```python
from build123d import *

# Parameters (mm, degrees)
SKETCH2_R               = 4.7625
BOSS_EXTRUDE1_DEPTH     = 75.565
CUT_EXTRUDE1_DEPTH      = 8.255
CUT_EXTRUDE1_DEPTH_BACK = 8.255
SKETCH3_OUTSIDE_W       = 26.878
SKETCH3_OUTSIDE_H       = 26.878
SKETCH3_OUTSIDE_R       = 4.1275


with BuildPart() as part:
    # Sketch2 → Boss-Extrude1 (new body)
    with BuildSketch(Plane(origin=(0, 0, 0), x_dir=(1, 0, 0), z_dir=(0, 1, 0))):
        with Locations(Location((0, 0, 0), (0, 0, 270))):
            Circle(SKETCH2_R)
    extrude(amount=BOSS_EXTRUDE1_DEPTH)

    # Sketch3 outside → Cut-Extrude1 (cut, two sides: drawn at the far end of the back side and taken through both)
    with BuildSketch(Plane(origin=(0, 37.7825, 0), x_dir=(1, 0, 0), z_dir=(0, 1, 0)).offset(-CUT_EXTRUDE1_DEPTH_BACK)):
        Rectangle(SKETCH3_OUTSIDE_W, SKETCH3_OUTSIDE_H)
        with Locations(Location((0, 0, 0), (0, 0, 270))):
            Circle(SKETCH3_OUTSIDE_R, mode=Mode.SUBTRACT)
    extrude(amount=CUT_EXTRUDE1_DEPTH + CUT_EXTRUDE1_DEPTH_BACK, mode=Mode.SUBTRACT)


solid = part.part
```
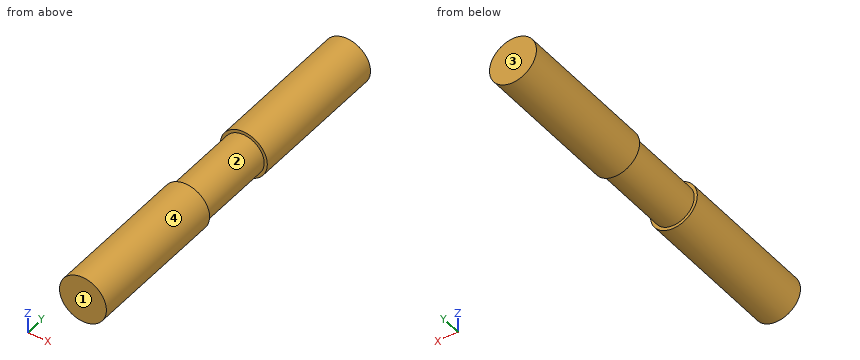
Geometry check sheet. Reference: the model listing, model coordinates, mm. Face numbers are marked on the shaded views. Give positions to 0.01 mm unless a question says otherwise; leave off trailing zeros. Loops run counter-clockwise (first coordinate to the right, second up) from the corner with the lowest first, then second, coordinate; pieces in that order, holes last. Notation, with made-up numbers: (51, -33.5) - (59, -33.5) arc R24 cw to (59, 2.5) - close; hole circle Ø1 at (66.25, 45.5). An arc over 180 degrees is marked (long way). Use CSV: the item, a comma, the result in double quotes. Start each with the question number.
Q1. Section check C-C, the plane y = 53. Record the cut outline in (x, z) (1 decimal), and give its area (3 significant figures).
Q2. Go/stop test with a flat-tipped pin: pin 1 Ø1.5 at (y, z) = (8, -2) entering from -X. Record where the tip stops, or that it passes through.
Q3. Release check for a two-part mould opening along Y. For the marked faces 1, 2, 3 and 4 record: +Y half, -Y half, draft (parallel to the pull), parting line (faces both ways), or undercut.
Q4. Section check B-B, the plane z = 0. Record the cut outline in (x, y) (1 decimal).
Q5. Scan lines: probe 1 along Y at (x, z) = (-3.75, 2) (1 decimal); probe 2 along Z at (x, y) = (-0.25, 5.5); probe 3 along Z at (x, y) = (-3.75, 62). Record each from-to range of solid material in increasing order. Write a range as from..to.
Q6. Section check A-A, the plane x = 0. Record the cut outline in (y, z) (1 decimal).
Findings below:
1,outline,"circle Ø9.5 at (0, 0)"
1,area,"71.3 mm^2"
2,pin 1,"stops at x = -4.6"
3,face 1,"-Y half"
3,face 2,"undercut"
3,face 3,"+Y half"
3,face 4,"draft"
4,outline,"(-4.8, 0) - (4.8, 0) - (4.8, 29.5) - (4.1, 29.5) - (4.1, 46) - (4.8, 46) - (4.8, 75.6) - (-4.8, 75.6) - (-4.8, 46) - (-4.1, 46) - (-4.1, 29.5) - (-4.8, 29.5) - close"
5,probe 1,"y = 0..29.5, 46..75.6"
5,probe 2,"z = -4.76..4.76"
5,probe 3,"z = -2.94..2.94"
6,outline,"(0, -4.8) - (29.5, -4.8) - (29.5, -4.1) - (46, -4.1) - (46, -4.8) - (75.6, -4.8) - (75.6, 4.8) - (46, 4.8) - (46, 4.1) - (29.5, 4.1) - (29.5, 4.8) - (0, 4.8) - close"
